The listing builds one solid part. Answer for the finished solid, in the listing's coordinates (mm). A direction names the side the tool comes from. Coordinates: 2 decimals unless noted, no trailing zeros. Write each loop counter-clockwise with the first axis right and the second up, starting at its lowest first coordinate (ties: lowest second). Pieces come first, ordered by that corner, then holes. Notation, with made-up numbers: M 80,3.5 L 98,3.5 A24 cw 98,28.5 Z; hole C 2.5,-21.5 d2. An arc over 180 degrees is marked long. Answer as CSV lines item,"result".
```python
from build123d import *

# Parameters (mm, degrees)
F0_W      = 127
F0_H      = 76.2
F1_DEPTH  = 82.55
F3_W      = 25.4
F3_H      = 73.025
F3_W_2    = 69.85
F4_DEPTH  = 80.9625
F6_DEPTH  = 127.001
F8_DEPTH  = 1.5875
F10_DEPTH = 1.5875
F11_W     = 50.8
F11_H     = 26.9875
F11_H_2   = 1.5875
F11_H_3   = 25.4
F12_DEPTH = 1.5875
F13_W     = 50.8
F13_H     = 1.5875
F14_DEPTH = 25.4
F15_R     = 3.3734375
F16_DEPTH = 1.5875
F17_R     = 3.3734375
F18_DEPTH = 1.5875


# Not quite as in the source:
# - a length typed as a fraction of an inch, garbled in the dataset ("3 / 203.2 mm" for 3/8 in), is restored


with BuildPart() as f1:
    # F0 (on Top) → F1 (new body)
    with BuildSketch(Plane.XY):
        Rectangle(F0_W, F0_H)
    extrude(amount=F1_DEPTH)

    # F3 (on face) → F4 (cut)
    with BuildSketch(Plane.XY.offset(82.55)):
        Polygon((-61.9125, 36.5125), (-61.9125, 0), (-61.9125, -36.5125), (-36.5125, -36.5125), (-36.5125, 36.5125), align=None)
        with Locations((49.2125, 0)):
            Rectangle(F3_W, F3_H)
        Rectangle(F3_W_2, F3_H)
    extrude(amount=-F4_DEPTH, mode=Mode.SUBTRACT)

    # F5 (on face) → F6 (cut, through all)
    with BuildSketch(Plane.YZ.offset(63.5)):
        with BuildLine():
            Line((12.7, 69.85), (12.7, 82.55))
            Line((12.7, 82.55), (0, 82.55))
            Line((0, 82.55), (-12.7, 82.55))
            Line((-12.7, 82.55), (-12.7, 69.85))
            ThreePointArc((-12.7, 69.85), (-8.9802561211, 60.8697438789), (0, 57.15))
            ThreePointArc((0, 57.15), (8.9802561211, 60.8697438789), (12.7, 69.85))
        make_face()
    extrude(amount=-F6_DEPTH, mode=Mode.SUBTRACT)

    # F7 (on face) → F8 (join)
    with BuildSketch(Plane.XZ.offset(38.1)):
        Polygon((-12.7, 0), (0, 0), (12.7, 0), (25.4, 0), (25.4, 107.95), (12.7, 107.95), (-12.7, 107.95), (-25.4, 107.95), (-25.4, 0), align=None)
    extrude(amount=F8_DEPTH)

    # F9 (on face) → F10 (join)
    with BuildSketch(Plane(origin=(0, 38.1, 0), x_dir=(-1, 0, 0), z_dir=(0, 1, 0))):
        Polygon((-12.7, 0), (0, 0), (12.7, 0), (25.4, 0), (25.4, 82.55), (-25.4, 82.55), (-25.4, 0), align=None)
        Polygon((-25.4, 82.55), (25.4, 82.55), (25.4, 107.95), (12.7, 107.95), (-12.7, 107.95), (-25.4, 107.95), align=None)
    extrude(amount=F10_DEPTH)

    # F11 (on face) → F12 (join)
    with BuildSketch(Plane.XY.offset(107.95)):
        with Locations((0, -51.59375)):
            Rectangle(F11_W, F11_H)
        with Locations((0, 38.89375)):
            Rectangle(F11_W, F11_H_2)
        with Locations((0, 52.3875)):
            Rectangle(F11_W, F11_H_3)
    extrude(amount=F12_DEPTH)

    # F13 (on face) → F14 (join)
    with BuildSketch(Plane(origin=(0, 0, 107.95), x_dir=(1, 0, 0), z_dir=(0, 0, -1))):
        with Locations((0, 64.29375)):
            Rectangle(F13_W, F13_H)
        with Locations((0, -64.29375)):
            Rectangle(F13_W, F13_H)
    extrude(amount=F14_DEPTH)

    # F15 (on face) → F16 (cut)
    with BuildSketch(Plane.XZ.offset(65.0875)):
        with Locations((12.7, 96.04375)):
            Circle(F15_R)
        with Locations((-12.7, 96.04375)):
            Circle(F15_R)
    extrude(amount=-F16_DEPTH, mode=Mode.SUBTRACT)

    # F17 (on face) → F18 (cut)
    with BuildSketch(Plane(origin=(0, 65.0875, 0), x_dir=(-1, 0, 0), z_dir=(0, 1, 0))):
        with Locations((12.7, 96.04375)):
            Circle(F17_R)
        with Locations((-12.7, 96.04375)):
            Circle(F17_R)
    extrude(amount=-F18_DEPTH, mode=Mode.SUBTRACT)


solid = f1.part
```
Q1. The mould has two halves that part along Z. Classify faces 1 (the flat face through (0, 1, 1.587)), 2 (the flat face through (-34.925, -1, 43)), 3 (the cylindrical face through (-13.43, -64.3, 92.75)): pulls with the +Z half, pulls with the -Z half, needs draft (parallel to the pull), parting line crosses it, or undercut.
Output:
face 1,"pulls with the +Z half"
face 2,"needs draft"
face 3,"undercut"
Q2. Find section D-D (z = 84.5). Give the vertices of the cut face in (x, y), and give its area (3 significant figures).
Output:
outline,"M -25.4,-65.09 L 25.4,-65.09 L 25.4,-63.5 L -25.4,-63.5 Z; M -25.4,-39.69 L 25.4,-39.69 L 25.4,-38.1 L -25.4,-38.1 Z; M -25.4,38.1 L 25.4,38.1 L 25.4,39.69 L -25.4,39.69 Z; M -25.4,63.5 L 25.4,63.5 L 25.4,65.09 L -25.4,65.09 Z"
area,"323 mm2"
Q3. Flat-ended cylindrical pins translate along their axes: pin 1 Ø12.5 at (x, y) = (-12.5, -21.5) entering from +Z; pin 2 Ø7.5 at (x, z) = (-55.5, 22.5) entering from +Y; pin 3 Ø21 at (x, z) = (-2.5, 55.5) entering from -Y. Find the tip coordinate at first contact, or state that the pin passes through.
Output:
pin 1,"z = 1.59"
pin 2,"y = 38.1"
pin 3,"y = -39.69"
Q4. For faces 4 (the flat face through (61.912, -1, 43)), 5 (the flat face through (0, 38.1, 96)), 6 (the flat face through (25.4, -39.5, 63.1)), 7 (the flat face through (0, 52, 107.95)), 8 (the flat face through (44, 38.1, 41)), determine the directions among +Z, -Z, +X, -X, +Y, -Y from which every point of the face is accessible in a straight line to the end or side of a thin tool.
Output:
face 4,"+Z"
face 5,"+Z, +X, -X"
face 6,"+Z, -Z, +X, -Y"
face 7,"-Z, +X, -X"
face 8,"+Z, -Z, +X, +Y"
Q5. Find section B-B (z = 27.5). Give the vertices of the cut face in (x, y) (1 decimal), and give its area (3 significant figures).
Output:
outline,"M -63.5,-38.1 L -25.4,-38.1 L -25.4,-39.7 L 25.4,-39.7 L 25.4,-38.1 L 63.5,-38.1 L 63.5,38.1 L 25.4,38.1 L 25.4,39.7 L -25.4,39.7 L -25.4,38.1 L -63.5,38.1 Z; hole M -61.9,-36.5 L -36.5,-36.5 L -36.5,36.5 L -61.9,36.5 Z; hole M -34.9,-36.5 L 34.9,-36.5 L 34.9,36.5 L -34.9,36.5 Z; hole M 36.5,-36.5 L 61.9,-36.5 L 61.9,36.5 L 36.5,36.5 Z"
area,"1,030 mm2"
Q6. Straight lines are drawn through the part: line 1 (X direction, y = 16, z = 68) (1 decimal); line 2 (Y direction, x = -5, z = 92); line 3 (Y direction, x = 42.5, z = 55). For each, find the intervals that lie inside material, in ascending order.
Output:
line 1,"-63.5 to -61.9, -36.5 to -34.9, 34.9 to 36.5, 61.9 to 63.5"
line 2,"-65.09 to -63.5, -39.69 to -38.1, 38.1 to 39.69, 63.5 to 65.09"
line 3,"-38.1 to -36.51, 36.51 to 38.1"
Q7. Find section A-A (x = -12.7). Give the vertices of the cut face in (y, z).
Output:
outline,"M -65.09,82.55 L -63.5,82.55 L -63.5,92.67 L -65.09,92.67 Z; M -65.09,99.42 L -63.5,99.42 L -63.5,107.95 L -39.69,107.95 L -39.69,0 L 39.69,0 L 39.69,107.95 L 63.5,107.95 L 63.5,99.42 L 65.09,99.42 L 65.09,109.54 L 38.1,109.54 L 38.1,82.55 L 36.51,82.55 L 36.51,1.59 L -36.51,1.59 L -36.51,82.55 L -38.1,82.55 L -38.1,109.54 L -65.09,109.54 Z; M 63.5,82.55 L 65.09,82.55 L 65.09,92.67 L 63.5,92.67 Z"
